Can you work these out from the model? Positions are in its coordinate system, mm. A direction names the side the tool comes from. Give positions to 0.01 mm unless a question says otherwise; leave off trailing zeros. Write each loop counter-clockwise with the first axis right and the second up, starting at its lowest first coordinate (ties: lowest second). Pieces come first, ordered by that corner, then holes. Notation, with made-up numbers: (-33, -17.5) -> (25, -17.5) arc R24 cw to (25, 15.5) -> close; hole circle Ø1 at (15, 65). An arc over 180 degrees is marked (long way). One line per item, written item: value.
from build123d import *
from OCP.BRepFilletAPI import BRepFilletAPI_MakeChamfer

# Parameters (mm, degrees)
EXTRUSION1_DEPTH        = 19.5
ESQUISSE3_R             = 2.12
ENL_V_MAT_EXTRU_1_DEPTH = 61.204754796
ESQUISSE4_R             = 6.8
EXTRUSION2_DEPTH        = 2
ESQUISSE5_R             = 3
EXTRUSION3_DEPTH        = 3.5
CHANFREIN1_SIZE         = 2
ESQUISSE6_W             = 4
ESQUISSE6_H             = 1.5
EXTRUSION4_DEPTH        = 2
CHANFREIN2_SIZE         = 1
CHANFREIN2_SIZE2        = 1.732050808
ESQUISSE8_W             = 4.087218226
ESQUISSE8_H             = 8
ESQUISSE8_W_2           = 1
ESQUISSE8_H_2           = 5
EXTRUSION5_DEPTH        = 2
CONG_2_R                = 0.5
CONG_3_R                = 0.3


with BuildPart() as part:
    # Esquisse1 → Extrusion1 (new body)
    with BuildSketch(Plane(origin=(0, 0, 0), x_dir=(1, 0, 0), z_dir=(0, 1, 0))):
        Polygon((0, 27.8), (-7.7, 27.8), (-7.7, 30.35), (0, 30.35), (0, 33.85), (2.5, 33.85), (6, 36.3), (40.5, 36.3), (40.5, 30.35), (48.2, 30.35), (48.2, 27.8), (40.5, 27.8), (40.5, 0), (0, 0), align=None)
    extrude(amount=EXTRUSION1_DEPTH)

    # Esquisse3 → Enlèv. mat.-Extru.1 (cut, through all)
    with BuildSketch(Plane(origin=(0, 0, -30.35), x_dir=(-1, 0, 0), z_dir=(0, 0, -1))):
        with Locations((3.7, 4)):
            Circle(ESQUISSE3_R)
        with Locations((3.7, 15.5)):
            Circle(ESQUISSE3_R)
        with Locations((-44.2, 15.5)):
            Circle(ESQUISSE3_R)
        with Locations((-44.2, 4)):
            Circle(ESQUISSE3_R)
    extrude(amount=-ENL_V_MAT_EXTRU_1_DEPTH, mode=Mode.SUBTRACT)

    # Esquisse4 → Extrusion2 (add)
    with BuildSketch(Plane(origin=(0, 0, -36.3), x_dir=(-1, 0, 0), z_dir=(0, 0, -1))):
        with Locations(Location((-30.75, 9.75, 0), (0, 0, 180))):
            Circle(ESQUISSE4_R)
    extrude(amount=EXTRUSION2_DEPTH)

    # Esquisse5 → Extrusion3 (add)
    with BuildSketch(Plane(origin=(0, 0, -38.3), x_dir=(-1, 0, 0), z_dir=(0, 0, -1))):
        with Locations((-30.75, 9.75)):
            Circle(ESQUISSE5_R)
    extrude(amount=EXTRUSION3_DEPTH)

    # Chanfrein1
    chanfrein1_edges = [part.edges().sort_by_distance(p)[0] for p in [
        (23.95, 9.75, -38.3),
    ]]
    chamfer(chanfrein1_edges, length=CHANFREIN1_SIZE - 0.0001)  # a hair under: the kernel refuses the full size

    # Esquisse6 → Extrusion4 (add)
    with BuildSketch(Plane(origin=(0, 0, -30.35), x_dir=(-1, 0, 0), z_dir=(0, 0, -1))):
        with Locations((-42.5, 9.75)):
            Rectangle(ESQUISSE6_W, ESQUISSE6_H)
        with Locations((2, 9.75)):
            Rectangle(ESQUISSE6_W, ESQUISSE6_H)
    extrude(amount=EXTRUSION4_DEPTH)

    # Chanfrein2: one chamfer whose edges measure the first distance from different faces: ONE call of the kernel's chamfer builder (chamfer() names one face for all edges)
    chanfrein2_edges_1 = [part.edges().sort_by_distance(p)[0] for p in [
        (-4, 9.75, -32.35),
    ]]
    chanfrein2_side_1 = [part.faces().sort_by_distance(p)[0] for p in [
        (-4, 9.75, -31.35),
    ]]
    chanfrein2_edges_2 = [part.edges().sort_by_distance(p)[0] for p in [
        (44.5, 9.75, -32.35),
    ]]
    chanfrein2_side_2 = [part.faces().sort_by_distance(p)[0] for p in [
        (44.5, 9.75, -31.35),
    ]]
    chanfrein2 = BRepFilletAPI_MakeChamfer(part.part.solid().wrapped)
    for e in chanfrein2_edges_1:
        chanfrein2.Add(CHANFREIN2_SIZE, CHANFREIN2_SIZE2, e.wrapped, chanfrein2_side_1[0].wrapped)  # the first distance lies on this face
    for e in chanfrein2_edges_2:
        chanfrein2.Add(CHANFREIN2_SIZE, CHANFREIN2_SIZE2, e.wrapped, chanfrein2_side_2[0].wrapped)  # the first distance lies on this face
    add(Compound.cast(chanfrein2.Shape()), mode=Mode.REPLACE)

    # Esquisse8 → Extrusion5 (add)
    with BuildSketch(Plane(origin=(40.5, 0, 0), x_dir=(0, 0, -1), z_dir=(1, 0, 0))):
        with Locations((2.543609113, 9.75)):
            Rectangle(ESQUISSE8_W, ESQUISSE8_H)
        with Locations((2.5, 9.75)):
            Rectangle(ESQUISSE8_W_2, ESQUISSE8_H_2, mode=Mode.SUBTRACT)
    extrude(amount=EXTRUSION5_DEPTH)

    # Congé2
    cong_2_edges = [part.edges().sort_by_distance(p)[0] for p in [
        (40.5, 19.5, -13.9),
        (0, 0, -32.1),
        (1.25, 0, -33.85),
        (4.25, 0, -35.075),
        (23.25, 0, -36.3),
        (40.5, 0, -33.325),
        (40.5, 0, -13.9),
        (20.25, 0, 0),
        (0, 0, -13.9),
        (0, 9.75, -33.85),
        (40.5, 9.75, -36.3),
        (40.5, 19.5, -33.325),
        (40.5, 9.75, 0),
        (0, 9.75, 0),
        (23.25, 19.5, -36.3),
        (4.25, 19.5, -35.075),
        (1.25, 19.5, -33.85),
        (0, 19.5, -32.1),
        (0, 19.5, -13.9),
        (20.25, 19.5, 0),
    ]]
    fillet(cong_2_edges, radius=CONG_2_R - 0.0001)  # a hair under: the kernel refuses the full size

    # Congé3
    cong_3_edges = [part.edges().sort_by_distance(p)[0] for p in [
        (42.5, 9.75, -0.5),
        (42.5, 5.75, -2.543609113),
        (42.5, 9.75, -4.587218226),
        (42.5, 13.75, -2.543609113),
        (41.5, 13.75, -0.5),
        (41.5, 5.75, -0.5),
        (41.5, 5.75, -4.587218226),
        (41.5, 13.75, -4.587218226),
    ]]
    fillet(cong_3_edges, radius=CONG_3_R)


solid = part.part
1) If we section it at C-C (y = 15.5): State how many separate pieces and enclosed holes the cut face has, and give its area (3 significant figures).
Answer list:
separate pieces: 3
enclosed holes: 0
area: 1,480 mm^2
2) Will these pins go through, and if not, where does the flat tip stop? pin 1 (1.5 mm diameter, centred on x = 37.5, y = 13.5, fed in from -Z); pin 2 (4 mm diameter, centred on x = 44.2, y = 15.5, fed in from +Z); pin 3 (0.6 mm diameter, centred on x = 42.5, z = -31.5, fed in from -Y); pin 4 (0.6 mm diameter, centred on x = 1.5, y = 6, fed in from -Z).
Answer list:
pin 1: stops at z = -36.3
pin 2: passes through
pin 3: stops at y = 9
pin 4: stops at z = -33.85
3) If we section it at A-A (z = -19.5): Write out the boundary of the cut face in (x, y).
Answer list:
outline: (0, 0.5) arc R0.5 ccw to (0.5, 0) -> (40, 0) arc R0.5 ccw to (40.5, 0.5) -> (40.5, 19) arc R0.5 ccw to (40, 19.5) -> (0.5, 19.5) arc R0.5 ccw to (0, 19) -> close
4) I need wall thicknesses on L1, parallel to Y at x = -3.7, z = -29; L2, parallel to X at y = 4.25, z = -4; L3, parallel to Z at x = 0.5, y = 18.75. Which ranges of each line are inside material? Lowest first, please.
Answer list:
L1: y = 0 to 1.88, 6.12 to 13.38, 17.62 to 19.5
L2: x = 0 to 40.5
L3: z = -33.85 to 0
5) We'd pull the mould along Z, two halves only. Please class faces 6 (the face through (41, 10, -2)), 7 (the face through (41, 10, -0.5)), 8 (the face through (0, 10, -14)): released by +Z, released by -Z, zero draft, split by the parting line, or undercut.
Answer list:
face 6: undercut
face 7: released by +Z
face 8: zero draft
6) If we section it at B-B (x = 18.5): Write out the boundary of the cut face in (y, z).
Answer list:
outline: (0, -35.8) arc R0.5 ccw to (0.5, -36.3) -> (19, -36.3) arc R0.5 ccw to (19.5, -35.8) -> (19.5, -0.5) arc R0.5 ccw to (19, 0) -> (0.5, 0) arc R0.5 ccw to (0, -0.5) -> close
7) For faces 1 (the face through (41, 13.75, -3)), 2 (the face through (-2, 9, -31)), 3 (the face through (1, 10, -33.85)), 4 (the face through (42.5, 9.8, -1.7)), 5 (the face through (33.747, 9.882, -40.025)), which set-ups out of +Z, -Z, +X, -X, +Y, -Y let a thin tool reach every point of the face, with its end or its side?
Answer list:
face 1: +Z, +X, +Y
face 2: -Z, -X, -Y
face 3: -Z, -X, +Y, -Y
face 4: +Z, +X, +Y, -Y
face 5: -Z
